from build123d import *

# Parameters (mm, degrees)
SKETCH1_R           = 1.5
BOSS_EXTRUDE1_DEPTH = 45.72
CUT_EXTRUDE1_DEPTH  = 25.4


with BuildPart() as part:
    # Sketch1 → Boss-Extrude1 (new body)
    with BuildSketch(Plane.XY):
        with BuildLine():
            add(Edge.make_bspline(
                [(8.677884321, 18.376352753), (9.611503438, 20.442753269), (9.364466551, 22.79145978)],
                knots=[4.222526815, 4.222526815, 4.222526815, 5.034979768, 5.034979768, 5.034979768], degree=2, weights=[1, 0.918618451, 1]))
            Line((8.677884321, 18.376352753), (5.066951203, 10.384192012))
            ThreePointArc((5.066951203, 10.384192012), (4.129783184, 9.29599528), (2.752240497, 8.89))
            Line((2.752240497, 8.89), (2.54, 8.89))
            ThreePointArc((2.54, 8.89), (0.743948776, 8.146051224), (0, 6.35))
            Line((0, 6.35), (0, 2.54))
            ThreePointArc((0, 2.54), (0.743948776, 0.743948776), (2.54, 0))
            Line((2.54, 0), (10.16, 0))
            ThreePointArc((10.16, 0), (11.956051224, 0.743948776), (12.7, 2.54))
            Line((12.7, 2.54), (12.7, 27.94))
            ThreePointArc((12.7, 27.94), (11.956051224, 29.736051224), (10.16, 30.48))
            Line((10.16, 30.48), (2.54, 30.48))
            ThreePointArc((2.54, 30.48), (0.743948776, 29.736051224), (0, 27.94))
            Line((0, 27.94), (0, 24.08))
            ThreePointArc((0, 24.08), (1.01383309, 22.739069096), (2.58032425, 23.349035215))
            ThreePointArc((2.58032425, 23.349035215), (2.620527336, 23.41287828), (2.661984223, 23.475914394))
            add(Edge.make_bspline(
                [(6.406345811, 26.98329616), (3.861791417, 27.243144961), (2.661984223, 23.475914394)],
                knots=[0, 0, 0, 1.248205539, 1.248205539, 1.248205539], degree=2, weights=[1, 0.81148776, 1]))
            add(Edge.make_bspline(
                [(9.364466551, 22.79145978), (8.950900204, 26.723447359), (6.406345811, 26.98329616)],
                knots=[5.034979768, 5.034979768, 5.034979768, 6.283185307, 6.283185307, 6.283185307], degree=2, weights=[1, 0.81148776, 1]))
        make_face()
        with Locations((4.965459901, 4.445)):
            Circle(SKETCH1_R, mode=Mode.SUBTRACT)
    extrude(amount=BOSS_EXTRUDE1_DEPTH)

    # Sketch2 → Cut-Extrude1 (cut)
    with BuildSketch(Plane(origin=(12.7, 0, 0), x_dir=(0, 0, -1), z_dir=(1, 0, 0))):
        with BuildLine():
            Line((-40.64, 0), (-5.08, 0))
            Line((-5.08, 0), (-5.08, 16.51))
            ThreePointArc((-5.08, 16.51), (-5.823948776, 18.306051224), (-7.62, 19.05))
            Line((-7.62, 19.05), (-38.1, 19.05))
            ThreePointArc((-38.1, 19.05), (-39.896051224, 18.306051224), (-40.64, 16.51))
            Line((-40.64, 16.51), (-40.64, 0))
        make_face()
    extrude(amount=-CUT_EXTRUDE1_DEPTH, mode=Mode.SUBTRACT)


solid = part.part
Could you check a few things on this model? Use its own coordinates, in mm. A direction names the side the tool comes from. Give positions to 0.01 mm unless a question says otherwise; leave off trailing zeros. Order: outer loops, then holes, each group sorted by start corner. A loop starts at its lowest first (then second) coordinate and runs counter-clockwise, first axis right, second up. Notation, with made-up numbers: (33.25, 61) -> (77.25, 61) arc R14 cw to (77.25, 70) -> close; hole circle Ø2 at (38.5, 49.5). An arc over 180 degrees is marked (long way). Return JSON: item names as keys, results as strings.
1. Imagine slicing it at A-A on x = 1.25. List the corners of the cut face in (y, z) for me, then the cut area to 3 significant figures.
Answer list:
{"outline": "(0.35, 0) -> (8.54, 0) -> (8.54, 5.08) -> (0.35, 5.08) -> close; (0.35, 40.64) -> (8.54, 40.64) -> (8.54, 45.72) -> (0.35, 45.72) -> close; (22.69, 0) -> (30.13, 0) -> (30.13, 45.72) -> (22.69, 45.72) -> close", "area": "423 mm2"}
2. I need wall thicknesses on line 1 (Z direction, x = 2.5, y = 8.5); line 2 (X direction, y = 25, z = 19); line 3 (X direction, y = 16.5, z = 44). Which ranges of each line are inside material? Lowest first, please. Write a range as from..to.
Answer list:
{"line 1": "z = 0..5.08, 40.64..45.72", "line 2": "x = 0..3.34, 8.77..12.7", "line 3": "x = 7.83..12.7"}
3. Imagine slicing it at B-B on y = 8. List the corners of the cut face in (x, z) for me, then the cut area to 3 significant figures.
Answer list:
{"outline": "(0.61, 0) -> (12.7, 0) -> (12.7, 5.08) -> (0.61, 5.08) -> close; (0.61, 40.64) -> (12.7, 40.64) -> (12.7, 45.72) -> (0.61, 45.72) -> close", "area": "123 mm2"}
4. On a 3-axis mill with a long thin cutter (end or side, diameter ignored), from which of +Z, -Z, +X, -X, +Y, -Y can I reach the whole of each face in a straight line? I mean faces 4 (the cylindrical face through (0.8, 8.2, 2.5)), 5 (the flat face through (8, 7, 40.64)), 6 (the cylindrical face through (0.99, 22.746, 22.54)). Say none if no direction works.
Answer list:
{"face 4": "+Z, -Z, -X", "face 5": "+X, -X, -Y", "face 6": "+Z, -Z"}
5. For pin 1 Ø4 at (x, y) = (3.5, 10.5) entering from +Z; pin 2 Ø1.1 at (x, z) = (10.5, 24) entering from -Y; pin 3 Ø1 at (x, z) = (1.5, 17) entering from +Y, each with a flat end and sliding along its axis, tell me the tip position at first contact or that it passes through.
Answer list:
{"pin 1": "stops at z = 45.72", "pin 2": "stops at y = 19.05", "pin 3": "stops at y = 30.42"}
6. Imagine slicing it at C-C on y = 16. List the corners of the cut face in (x, z) for me, then the cut area to 3 significant figures.
Answer list:
{"outline": "(7.6, 0) -> (12.7, 0) -> (12.7, 5.08) -> (7.6, 5.08) -> close; (7.6, 40.64) -> (12.7, 40.64) -> (12.7, 45.72) -> (7.6, 45.72) -> close", "area": "51.8 mm2"}
7. Thinking about a two-plate mould opening in X: for faces 1 (the cylindrical face through (0.724, 0.764, 2.504)), 2 (the flat face through (6, 0, 43)), 3 (the cylindrical face through (6.396, 4.896, 43.144)), which applies, pulls with the +X half, pulls with the -X half, needs draft (parallel to the pull), parting line crosses it, or undercut?
Answer list:
{"face 1": "pulls with the -X half", "face 2": "needs draft", "face 3": "undercut"}
